Autodesk Inventor part; units mm, degrees
ref_plane "YZ Plane" through (0, 0, 0) normal (1, 0, 0) x (0, 1, 0)
ref_plane "XZ Plane" through (0, 0, 0) normal (0, 1, 0) x (-1, 0, 0)
ref_plane "XY Plane" through (0, 0, 0) normal (0, 0, 1) x (1, 0, 0)
sketch "Эскиз1" plane through (0, 0, 0) normal (0, 1, 0) x (-1, 0, 0)
  circle A0 centre (0, 0) radius 14
  circle A1 centre (0, 0) radius 24 construction
  circle A2 centre (0, 0) radius 55
  circle A3 centre (23.9999, 0) radius 5
  circle A4 centre (12, 20.7845) radius 5
  circle A5 centre (-12, 20.7845) radius 5
  circle A6 centre (-23.9999, 0) radius 5
  circle A7 centre (-12, -20.7845) radius 5
  circle A8 centre (12, -20.7845) radius 5
  line L0 (-54.9999, -55) -> (54.9999, -55)
  line L1 (54.9999, -55) -> (54.9999, 55)
  line L2 (54.9999, 55) -> (-54.9999, 55)
  line L3 (-54.9999, 55) -> (-54.9999, -55)
  line L4 (-54.9999, -55) -> (54.9999, 55) construction
  line L5 (54.9999, -55) -> (-54.9999, 55) construction
  dimension "d0" = 28
  dimension "d1" = 48
  dimension "d2" = 110
  dimension "d3" = 10
  dimension "d6" = 360
extrude "Выдавливание1" add sketch "Эскиз1" along normal blind 10
sketch "Эскиз2" plane through (0, 10, 0) normal (0, 1, 0) x (1, 0, 0)
  circle A0 centre (0, 0) radius 14
  circle A1 centre (0, 37.5) radius 12.5
  circle A2 centre (-32.476, 18.75) radius 12.5
  circle A3 centre (-32.476, -18.75) radius 12.5
  circle A4 centre (0, -37.5) radius 12.5
  circle A5 centre (32.476, -18.75) radius 12.5
  circle A6 centre (32.476, 18.75) radius 12.5
  dimension "d10" = 25
  dimension "d13" = 360
  dimension "d19" = 37.5
extrude "Выдавливание2" cut sketch "Эскиз2" against normal blind 10 contours A1 | A2 | A3 | A4 | A5 | A6
sketch "Эскиз3" plane through (0, 10, 0) normal (0, 1, 0) x (1, 0, 0)
  circle A0 centre (0, 0) radius 55
  circle A1 centre (0, 0) radius 14
  circle A2 centre (0, 18) radius 2.5
  circle A3 centre (-15.5885, 9) radius 2.5
  circle A4 centre (-15.5885, -9) radius 2.5
  circle A5 centre (0, -18) radius 2.5
  circle A6 centre (15.5885, -9) radius 2.5
  circle A7 centre (15.5885, 9) radius 2.5
  point P0 (44.976, 18.75)
  point P1 (12.5, 37.5)
  dimension "d20" = 5
  dimension "d22" = 18
  dimension "d25" = 360
extrude "Выдавливание3" cut sketch "Эскиз3" against normal blind 10 contours A2 | A3 | A4 | A5 | A6 | A7
sketch "Эскиз4" plane through (0, 10, 0) normal (0, 1, 0) x (1, 0, 0)
  circle A0 centre (0, 0) radius 14
  circle A1 centre (50, 0) radius 3
  circle A2 centre (25, 43.3013) radius 3
  circle A3 centre (-25, 43.3013) radius 3
  circle A4 centre (-50, 0) radius 3
  circle A5 centre (-25, -43.3013) radius 3
  circle A6 centre (25, -43.3013) radius 3
  dimension "d29" = 6
  dimension "d30" = 50
  dimension "d33" = 360
extrude "Выдавливание4" cut sketch "Эскиз4" against normal blind 10 contours A1 | A2 | A3 | A4 | A5 | A6
properties part number "Статор цевков"
The listing builds one solid part. Answer for the finished solid, in the listing's coordinates (mm). Round coordinates to 2 decimals unless told otherwise and drop trailing zeros. Order: outer loops, then holes, each group sorted by start corner. A loop starts at its lowest first (then second) coordinate and runs counter-clockwise, first axis right, second up. Notation, with made-up numbers: (81, 68) -> (123, 68) arc R21 ccw to (123, 91) -> close; hole circle Ø7 at (29.25, -10.75). An arc over 180 degrees is marked (long way). Answer as CSV lines item,"result". Start each with the question number.
(1) A flat-ended cylindrical pin translates along its axis: pin 1 Ø20 at (x, z) = (-32.476, -18.75) entering from -Y. Find the tip coordinate at first contact, or state that the pin passes through.
(2) Find the intervals of material crossed by probe 1 along X at (y, z) = (2.75, -30); probe 2 along X at (y, z) = (4.5, -12); probe 3 along Z at (x, y) = (39.5, 4.5), in increasing order. Write a range as from..to.
(3) The part is cut by section C-C (x = 0). Determine the outline of the cut face in (y, z), then the cut area to 3 significant figures.
(4) The part is cut by section A-A (z = -37.5). Determine the outline of the cut face in (x, y).
(5) The part is cut by section B-B (x = 50). Determine the outline of the cut face in (y, z), then the cut area to 3 significant figures.
(6) For a pull along X with two mould halves and no side action, classify faces 1 (the face through (-0.33, 5.07, -20.48)), 2 (the face through (-55, 5, -1)), 3 (the face through (55, 5, 1)) as +X half, -X half, draft (parallel to the pull), parting line (faces both ways), or undercut.
(7) The part is cut by section D-D (y = 2.25). Count the separate pieces of the cut face and the enclosed holes in it, then the cut area to 3 significant figures.
Evaluation:
1,pin 1,"through"
2,probe 1,"-55..-37.92, -27.03..-10, 10..27.03, 37.92..55"
2,probe 2,"-55..-43, -21.96..-7.21, 7.21..21.96, 43..55"
2,probe 3,"-55..-29.09, -8.41..8.41, 29.09..55"
3,outline,"(0, -55) -> (10, -55) -> (10, -50) -> (0, -50) -> close; (0, -25) -> (10, -25) -> (10, -20.5) -> (0, -20.5) -> close; (0, -15.5) -> (10, -15.5) -> (10, -14) -> (0, -14) -> close; (0, 14) -> (10, 14) -> (10, 15.5) -> (0, 15.5) -> close; (0, 20.5) -> (10, 20.5) -> (10, 25) -> (0, 25) -> close; (0, 50) -> (10, 50) -> (10, 55) -> (0, 55) -> close"
3,area,"220 mm²"
4,outline,"(-55, 0) -> (-12.5, 0) -> (-12.5, 10) -> (-55, 10) -> close; (12.5, 0) -> (55, 0) -> (55, 10) -> (12.5, 10) -> close"
5,outline,"(0, -55) -> (10, -55) -> (10, -3) -> (0, -3) -> close; (0, 3) -> (10, 3) -> (10, 55) -> (0, 55) -> close"
5,area,"1,040 mm²"
6,face 1,"undercut"
6,face 2,"-X half"
6,face 3,"+X half"
7,separate pieces,"1"
7,enclosed holes,"25"
7,area,"7,780 mm²"
